from build123d import *

# Parameters (mm, degrees)
BOSS_EXTRUDE1_DEPTH = 4.826
FILLET1_R           = 25.4
LPATTERN1_COUNT     = 22
LPATTERN1_PITCH     = 12.7
CIRPATTERN1_COUNT   = 4
CHAMFER1_SIZE       = 0.396875


with BuildPart() as part:
    # Sketch1 → Boss-Extrude1 (new body)
    with BuildSketch(Plane.XY):
        with BuildLine():
            Line((15.875, 27.49630657), (15.875, 304.8))
            ThreePointArc((15.875, 304.8), (0, 320.675), (-15.875, 304.8))
            Line((-15.875, 304.8), (-15.875, 27.49630657))
            ThreePointArc((-15.875, 27.49630657), (0, -31.75), (15.875, 27.49630657))
        make_face()
    extrude(amount=BOSS_EXTRUDE1_DEPTH)

    # Fillet1
    fillet1_edges = [part.edges().sort_by_distance(p)[0] for p in [
        (-15.875, 27.49630657, 2.413),
        (15.875, 27.49630657, 2.413),
    ]]
    fillet(fillet1_edges, radius=FILLET1_R)

    # Sketch3 → #8-32 Tapped Hole1 (revolve, cut)
    with BuildSketch(Plane(origin=(0, 304.8, 4.826), x_dir=(0, -1, 0), z_dir=(1, 0, 0))):
        Polygon((0, 0), (0, 11.705806461), (1.7272, 10.668), (1.7272, 0), align=None)
    f_8_32_tapped_hole1 = revolve(axis=Axis((0, 304.8, 11.176), (0, 0, -1)), mode=Mode.SUBTRACT)

    # LPattern1: #8-32 Tapped Hole1 ×22
    with Locations(*[(0, -i * LPATTERN1_PITCH, 0) for i in range(1, LPATTERN1_COUNT)]):
        add(f_8_32_tapped_hole1, mode=Mode.SUBTRACT)

    # Sketch7 → CSK for M8 SFHCS1 (revolve, cut)
    with BuildSketch(Plane(origin=(0, -20.9999961, 4.826), x_dir=(0, -1, 0), z_dir=(1, 0, 0))):
        Polygon((0, 0), (0, 28.103872786), (4.5, 25.4), (4.5, 4.714), (9.214, 0), align=None)
    csk_for_m8_sfhcs1 = revolve(axis=Axis((0, -20.9999961, 11.176), (0, 0, -1)), mode=Mode.SUBTRACT)

    # CirPattern1: CSK for M8 SFHCS1 ×4 about axis
    cirpattern1_axis = Axis((0, 0, 0), (0, 0, 1))
    for i in range(1, CIRPATTERN1_COUNT):
        add(csk_for_m8_sfhcs1.rotate(cirpattern1_axis, i * 360 / CIRPATTERN1_COUNT), mode=Mode.SUBTRACT)

    # Chamfer1
    chamfer1_edges = [part.edges().sort_by_distance(p)[0] for p in [
        (0, 320.675, 4.826),
        (-15.875, 172.164215612, 4.826),
        (0, -31.75, 0),
        (0, -31.75, 4.826),
        (15.875, 172.164215612, 0),
        (15.875, 172.164215612, 4.826),
        (-17.704797531, 30.062410119, 0),
        (-17.704797531, 30.062410119, 4.826),
        (17.704797531, 30.062410119, 0),
        (17.704797531, 30.062410119, 4.826),
        (-15.875, 172.164215612, 0),
        (0, 320.675, 0),
    ]]
    chamfer(chamfer1_edges, length=CHAMFER1_SIZE)


solid = part.part
Design review of the part built by this model. Coordinates are the model's own, in mm. Coordinates: 2 decimals unless noted, no trailing zeros. Order: outer loops, then holes, each group sorted by start corner. A loop starts at its lowest first (then second) coordinate and runs counter-clockwise, first axis right, second up. Notation, with made-up numbers: (-15, 25) -> (19, 25) arc R22 cw to (19, 64) -> close; hole circle Ø8 at (32.5, 31). An arc over 180 degrees is marked (long way). Use one line per item in the form item = value. Start each with the question number.
(1) Add section B-B on z = 3.3. Give the number of separate pieces and of enclosed holes in the cut face, plus the area to 3 significant figures.
(2) For probe 1 along X at (y, z) = (279.4, 3.85) (3 decimals); probe 2 along X at (y, z) = (22.5, 3); probe 3 along Z at (x, y) = (-15.5, 291.5), list the stretches that pass through material, from the lowest coordinate up.
(3) Insertion check: pin 1 (1.5 mm diameter, centred on x = -9.5, z = 2.5, fed in from -Y); pin 2 (1 mm diameter, centred on y = 165.5, z = 1, fed in from -X) (3 decimals); pin 3 (14.5 mm diameter, centred on x = -21, y = 0, fed in from +Z); pin 4 (4 mm diameter, centred on x = 0, y = 241.3, fed in from +Z). Each pin has a flat end and moves straight along its axis. Give the tip position at first contact, or say it passes through.
(4) Add section A-A on y = 157. State the section outline as (x, z) points (3 decimals).
Answer block:
q1.separate_pieces = 1
q1.enclosed_holes = 26
q1.area = 11,400 mm²
q2.probe_1 = -15.875 to -1.727, 1.727 to 15.875
q2.probe_2 = -22.43 to -7.23, 7.23 to 22.43
q2.probe_3 = 0.02 to 4.8
q3.pin_1 = -30.52
q3.pin_2 = -15.875
q3.pin_3 = 2.86
q3.pin_4 = 4.83
q4.outline = (-15.875, 0.397) -> (-15.478, 0) -> (15.478, 0) -> (15.875, 0.397) -> (15.875, 4.429) -> (15.478, 4.826) -> (-15.478, 4.826) -> (-15.875, 4.429) -> close
